```python
from build123d import *

# Parameters (mm, degrees)
F2_R     = 3
F4_DEPTH = 20
F5_DEPTH = 20
F6_R     = 1.5
F7_DEPTH = 1.5
F8_R     = 0.75
F9_DEPTH = 55.5010001


with BuildPart() as f1:
    # F0 (on Top) → F1 (revolve)
    with BuildSketch(Plane.XY):
        with BuildLine():
            Line((-13.25, 0), (0, 0))
            Line((0, 0), (0, 37))
            Line((0, 37), (-1.5, 37))
            Line((-1.5, 37), (-1.5, 16.6235913226))
            ThreePointArc((-1.5, 16.6235913226), (-6.4401709177, 12.3947665973), (-11.3803418353, 16.6235913226))
            Line((-11.3803418353, 16.6235913226), (-11.4607692348, 17.1388115494))
            ThreePointArc((-11.4607692348, 17.1388115494), (-12.4196143352, 17.8973036522), (-13.25, 17))
            Line((-13.25, 17), (-13.25, 0))
        make_face()
    revolve(axis=Axis((0, 18.5, 0), (0, -1, 0)))

    # F2
    f2_edges = [f1.edges().sort_by_distance(p)[0] for p in [
        (1.5, 16.623591, 0),
    ]]
    fillet(f2_edges, radius=F2_R)

    # F3 (on face) → F4 (join)
    with BuildSketch(Plane.XZ):
        with BuildLine():
            Line((-12.2703911918, 5), (-38.25, 5))
            Line((-38.25, 5), (-38.25, -5))
            Line((-38.25, -5), (-12.2703911918, -5))
            ThreePointArc((-12.2703911918, -5), (-13.25, 0), (-12.2703911918, 5))
        make_face()
        with BuildLine():
            Line((12.2703911918, 5), (-12.2703911918, 5))
            ThreePointArc((-12.2703911918, 5), (-13.25, 0), (-12.2703911918, -5))
            Line((-12.2703911918, -5), (12.2703911918, -5))
            ThreePointArc((12.2703911918, -5), (13.0027916866, -2.5475298535), (13.25, 0))
            ThreePointArc((13.25, 0), (13.0027916866, 2.5475298535), (12.2703911918, 5))
        make_face()
        with BuildLine():
            Line((38.25, 5), (12.2703911918, 5))
            ThreePointArc((12.2703911918, 5), (13.0027916866, 2.5475298535), (13.25, 0))
            ThreePointArc((13.25, 0), (13.0027916866, -2.5475298535), (12.2703911918, -5))
            Line((12.2703911918, -5), (38.25, -5))
            Line((38.25, -5), (38.25, 5))
        make_face()
    extrude(amount=F4_DEPTH)

    # F5 (add): faces of the model
    f5_faces = [f1.faces().sort_by_distance(p)[0] for p in [
        (0, 0, 8.4077666552),
        (0, 0, -8.4077666552),
    ]]
    extrude(f5_faces, amount=F5_DEPTH)

    # F6 (on face) → F7 (cut)
    with BuildSketch(Plane(origin=(0, 37, 0), x_dir=(-1, 0, 0), z_dir=(0, 1, 0))):
        Circle(F6_R)
    extrude(amount=-F7_DEPTH, mode=Mode.SUBTRACT)

    # F8 (on face) → F9 (cut, through all)
    with BuildSketch(Plane.XZ.offset(20)):
        with Locations((-6.3117844984, 0)):
            Circle(F8_R)
    extrude(amount=-F9_DEPTH, mode=Mode.SUBTRACT)


solid = f1.part
```
Can you work these out from the model? Positions are in its coordinate system, mm. A direction names the side the tool comes from. Round coordinates to 2 decimals unless told otherwise and drop trailing zeros. Order: outer loops, then holes, each group sorted by start corner. A loop starts at its lowest first (then second) coordinate and runs counter-clockwise, first axis right, second up. Notation, with made-up numbers: (-38, 86.25) -> (-1, 86.25) arc R33 ccw to (-1, 118.25) -> close; hole circle Ø9 at (84.25, 51). An arc over 180 degrees is marked (long way). Return JSON: item names as keys, results as strings. Group by question number.
1. We'd pull the mould along Z, two halves only. Please class faces 4 (the face through (-25, 0, 0)), 5 (the face through (-7.06, -3.99, 0.03)), 6 (the face through (25, -10, 5)): released by +Z, released by -Z, zero draft, split by the parting line, or undercut.
2. Will these pins go through, and if not, where does the flat tip stop? pin 1 (8 mm diameter, centred on x = -7, y = 11.5, fed in from -Z); pin 2 (4 mm diameter, centred on y = 7.5, z = 6, fed in from +X); pin 3 (6 mm diameter, centred on x = -25, y = -7, fed in from -Z).
3. If we section it at A-A, the plane y = -14: Write out the boundary of the cut face in (x, z), then the cut area to 3 significant figures.
4. If we section it at B-B, the plane y = 29.5: Write out the boundary of the cut face in (x, z), then the cut area to 3 significant figures.
5. If we section it at C-C, the plane x = 24: Write out the boundary of the cut face in (y, z), then the cut area to 3 significant figures.
6. I need wall thicknesses on line 1 (X direction, y = -7, z = 0); line 2 (Z direction, x = -1.5, y = 13.5); line 3 (Z direction, x = 18, y = -7). Which ranges of each line are inside material? Lowest first, please. Write a range as [from, to].
7. Which directions (+Z, -Z, +X, -X, +Y, -Y) give clear straight access to the entire face, cutting with the end or side of a thin tool? Please do faces 1 (the face through (-25, -10, 5)), 2 (the face through (-1.43, 26.07, -0.45)), 3 (the face through (-25, -10, -5)).
Output values:
{
 "1": {"face 4": "zero draft", "face 5": "undercut", "face 6": "released by +Z"},
 "2": {"pin 1": "z = -12.91", "pin 2": "x = 12.63", "pin 3": "z = -5"},
 "3": {"outline": "(-38.25, -5) -> (-12.27, -5) arc R13.25 ccw to (12.27, -5) -> (38.25, -5) -> (38.25, 5) -> (12.27, 5) arc R13.25 ccw to (-12.27, 5) -> (-38.25, 5) -> close; hole circle Ø1.5 at (-6.31, 0)", "area": "1,060 mm²"},
 "4": {"outline": "circle Ø3 at (0, 0)", "area": "7.07 mm²"},
 "5": {"outline": "(-20, -5) -> (0, -5) -> (0, 5) -> (-20, 5) -> close", "area": "200 mm²"},
 "6": {"line 1": "[-38.25, -7.06], [-5.56, 38.25]", "line 2": "[-13.16, -9.46], [-2.94, 2.94], [9.46, 13.16]", "line 3": "[-5, 5]"},
 "7": {"face 1": "+Z, -X, +Y, -Y", "face 2": "+Y", "face 3": "-Z, -X, +Y, -Y"}
}
